from build123d import *

# Parameters (mm, degrees)
SKETCH1_W           = 395.409928
SKETCH1_H           = 228.6
BOSS_EXTRUDE1_DEPTH = 3.175
CUT_EXTRUDE1_DEPTH  = 3.175
BOSS_EXTRUDE2_REACH = 458.746
BOSS_EXTRUDE3_DEPTH = 50.165
BOSS_EXTRUDE5_REACH = 448.763


with BuildPart() as part:
    # Sketch1 → Boss-Extrude1 (new body)
    with BuildSketch(Plane(origin=(0, 0, 0), x_dir=(1, 0, 0), z_dir=(0, 1, 0))):
        with Locations((197.704964, 114.3)):
            Rectangle(SKETCH1_W, SKETCH1_H)
    extrude(amount=BOSS_EXTRUDE1_DEPTH)

    # Sketch2 → Cut-Extrude1 (cut)
    with BuildSketch(Plane(origin=(0, 3.175, 0), x_dir=(1, 0, 0), z_dir=(0, 1, 0))):
        Polygon((0, 0), (395.409928, 71.795894), (395.409928, 0), align=None)
    extrude(amount=-CUT_EXTRUDE1_DEPTH, mode=Mode.SUBTRACT)

    # Boss-Extrude2: up to this plane
    boss_extrude2_end = Plane(origin=(0, 0, 0), z_dir=(-0.17865222161961358, 0, -0.9839122845611679))
    # Sketch3 → Boss-Extrude2 (add, up to the surface)
    with BuildSketch(Plane(origin=(0, 0, -228.6), x_dir=(-1, 0, 0), z_dir=(0, 0, -1)), mode=Mode.PRIVATE) as boss_extrude2_sk1:
        Polygon((-395.409928, 3.175), (-408.296023119, -31.327136928), (-405.32170097, -32.438007197), (-392.020710392, 3.175), align=None)
    boss_extrude2_tool1 = split(extrude(boss_extrude2_sk1.sketch, amount=-BOSS_EXTRUDE2_REACH, mode=Mode.PRIVATE), bisect_by=boss_extrude2_end, keep=Keep.BOTH, mode=Mode.PRIVATE)
    add(boss_extrude2_tool1.solids().sort_by_distance((400.253689, -14.355253, -228.6))[0])

    # Sketch4 → Boss-Extrude3 (add)
    with BuildSketch(Plane(origin=(0, 0, -228.6), x_dir=(-1, 0, 0), z_dir=(0, 0, -1))):
        Polygon((0, 0), (11.108702689, 29.743221489), (8.13438054, 30.854091758), (-3.389217608, 0), align=None)
    extrude(amount=-BOSS_EXTRUDE3_DEPTH)

    # Boss-Extrude5: up to this plane
    boss_extrude5_end = Plane(origin=(0, 0, 0), z_dir=(-0.17865222161961358, 0, -0.9839122845611679))
    # Sketch6 → Boss-Extrude5 (add, up to the surface)
    with BuildSketch(Plane.XY.offset(-178.435), mode=Mode.PRIVATE) as boss_extrude5_sk1:
        Polygon((0, 3.175), (-29.743221489, -7.933702689), (-28.63235122, -10.908024838), (9.074529477, 3.175), align=None)
    boss_extrude5_tool1 = split(extrude(boss_extrude5_sk1.sketch, amount=BOSS_EXTRUDE5_REACH, mode=Mode.PRIVATE), bisect_by=boss_extrude5_end, keep=Keep.BOTH, mode=Mode.PRIVATE)
    add(boss_extrude5_tool1.solids().sort_by_distance((-12.225047, -3.152196, -178.435))[0])


solid = part.part
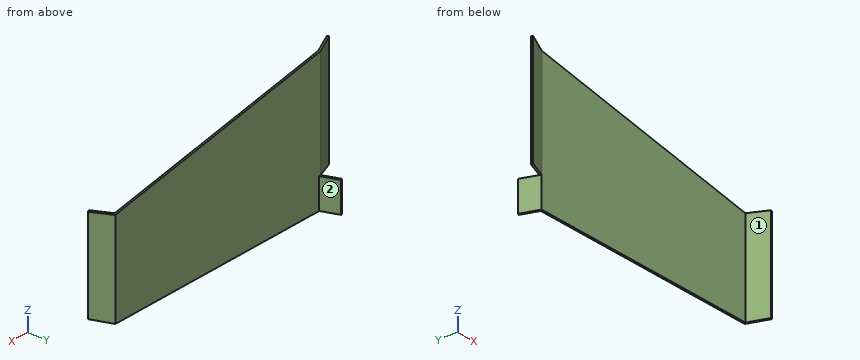
CAD build for the part. Positions are in the model's coordinates, mm. Face numbers are marked on the shaded views. A direction names the side the tool comes from. Round coordinates to 2 decimals unless told otherwise and drop trailing zeros. Loops run counter-clockwise (first coordinate to the right, second up) from the corner with the lowest first, then second, coordinate; pieces in that order, holes last.
(1) Wall check: line 1 along Y through (x, z) = (120.5, -111.5) (3 decimals); line 2 along X through (y, z) = (-21.5, -185); line 3 along X through (y, z) = (26, -196). Give the ranges that are in metal, low to high.
(2) Cut at B-B (z = -130). Give the cut face in (x, y) (3 decimals).
(3) Cut at D-D (y = -20). Give the cut face in (x, z).
(4) Cut at C-C (x = 370). Give the cut face in (y, z) (3 decimals).
(5) Cut at A-A (z = -184). Give the cut face in (x, y) (3 decimals).
(6) Which spindle directions (+Z, -Z, +X, -X, +Y, -Y) get a long thin tool onto all of the face, cutting with end or side? Do the marked faces 1 and 2. Say none if no direction does.
(7) Drop flat-ended pins along their axis: pin 1 (1 mm diameter, centred on x = 86.5, z = -70.5, fed in from +Y) (3 decimals); pin 2 (6 mm diameter, centred on x = 292, y = 7.5, fed in from +Z); pin 3 (10.5 mm diameter, centred on x = -3, y = 12.5, fed in from +Z) (3 decimals); pin 4 (11 mm diameter, centred on x = -20.5, y = -5, fed in from -Z) (3 decimals). Give the stop position or say it passes through.
Findings below:
1. line 1: y = 0 to 3.175
1. line 2: x = 401.24 to 404.63
1. line 3: x = -9.71 to -6.32
2. outline: (-29.743, -7.934) - (-28.632, -10.908) - (0.574, 0) - (393.207, 0) - (405.322, -32.438) - (408.296, -31.327) - (395.41, 3.175) - (0, 3.175) - close
3. outline: (400.68, -228.6) - (404.07, -228.6) - (404.07, -73.37) - (400.68, -72.75) - close
4. outline: (0, -228.6) - (3.175, -228.6) - (3.175, -67.182) - (0, -67.182) - close
5. outline: (-11.109, 29.743) - (0, 0) - (393.207, 0) - (405.322, -32.438) - (408.296, -31.327) - (395.41, 3.175) - (2.203, 3.175) - (-8.134, 30.854) - close
6. face 1: +Z, -Z, -Y
6. face 2: +Z, -Z, +X, +Y
7. pin 1: stops at y = 3.175
7. pin 2: passes through
7. pin 3: stops at z = -178.435
7. pin 4: stops at z = -178.435
